Autodesk Inventor part; units mm, degrees
ref_plane "YZ Plane" through (0, 0, 0) normal (1, 0, 0) x (0, 1, 0)
ref_plane "XZ Plane" through (0, 0, 0) normal (0, 1, 0) x (-1, 0, 0)
ref_plane "XY Plane" through (0, 0, 0) normal (0, 0, 1) x (1, 0, 0)
sketch "Sketch2" plane through (0, 0, 0) normal (0, 0, 1) x (1, 0, 0)
  circle A0 centre (0, 0) radius 2.5
  circle A1 centre (0, 0) radius 6
  dimension "d12" = 5
  dimension "d13" = 12
extrude "Extrusion1" add sketch "Sketch2" along normal blind 2.5
sketch "Sketch3" plane through (0, 0, 2.5) normal (0, 0, 1) x (1, 0, 0)
  circle A0 centre (0, 0) radius 2.5
  circle A1 centre (0, 0) radius 6
  line L0 (0, 0) -> (0, -18.3723) construction
  circle A2 centre (0, -17) radius 1.5
  circle A3 centre (0, -9) radius 1.25
  line L1 (3, -5.1962) -> (3, -17)
  line L2 (-3, -17) -> (-3, -5.1962)
  line L3 (5.4814, -17) -> (-5.6867, -17) construction
  arc A4 (-3, -17) -> (3, -17) centre (0, -17) ccw
  dimension "d16" = 3
  dimension "d17" = 2.5
  dimension "d18" = 9
  dimension "d19" = 17
  dimension "d20" = 3
  dimension "d21" = 3
extrude "Extrusion2" add sketch "Sketch3" against normal blind 2.5 contours A1 L1 A4 L2
pattern_circular "Circular Pattern1" count 4 over 360 about axis through (0, 0, 0) along (0, 0, 1) of "Extrusion2"
chamfer "Chamfer1" distance 0.6 angle 45 4 edges at (-1.5, -17, 2.5) (17, -1.5, 2.5) (-17, 1.5, 2.5) (1.5, 17, 2.5)
equation "\"d21\" = d20"
properties part number "HK 2830 mounting plate"
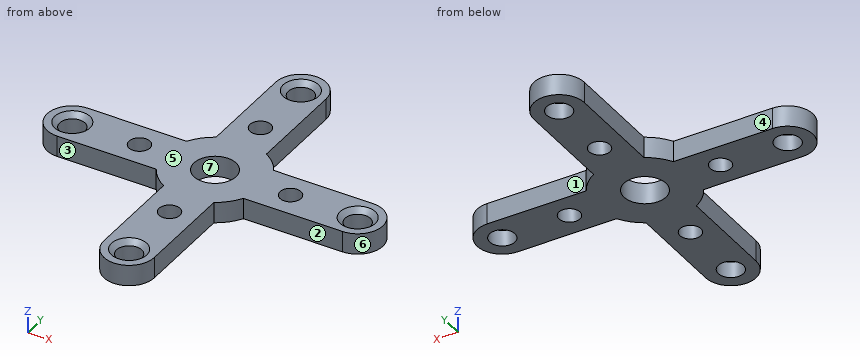
For this review, take the finished solid that the model builds, in its own axes (mm). Face numbers are marked on the shaded views. A direction names the side the tool comes from. Round coordinates to 2 decimals unless told otherwise and drop trailing zeros. Loops run counter-clockwise (first coordinate to the right, second up) from the corner with the lowest first, then second, coordinate; pieces in that order, holes last. Notation, with made-up numbers: (30.5, 20) - (78.5, 20) arc R20 ccw to (78.5, 28) - close; hole circle Ø5 at (25.5, -22). An arc over 180 degrees is marked (long way). Put each result on its own line as item: value. Start each with the question number.
1. For probe 1 along Y at (x, z) = (0, 0.65); probe 2 along Y at (x, z) = (17, 1.5), list the stretches that pass through material, from the lowest coordinate up. Write a range as [from, to].
2. Insertion check: P1, Ø1.2, axis at x = -11, z = 1.5, coming from the -Y side; P2, Ø1.2, axis at y = -11.5, z = 1.5, coming from the +X side. Each pin has a flat end and moves straight along its axis. Give the tip position at first contact, or say it passes through.
3. Mouldability with a two-part tool opening along Y and no side actions: class the marked faces 5, 6 and 7 as +Y half, -Y half, draft (parallel to the pull), parting line (faces both ways), or undercut.
4. Consider section C-C on y = -9. State the section outline as (x, z) points.
5. Consider section A-A on y = 0. State the section outline as (x, z) points.
6. For the marked faces 1, 2, 3 and 4, list the 3-axis set-ups (+Z, -Z, +X, -X, +Y, -Y) from which the entire face can be reached by the end or side of a thin tool; tool diameter is ignored.
Result sheet:
1. probe 1: [-20, -18.5], [-15.5, -10.25], [-7.75, -2.5], [2.5, 7.75], [10.25, 15.5], [18.5, 20]
1. probe 2: [-3, -1.5], [1.5, 3]
2. P1: y = -3
2. P2: x = 3
3. face 5: draft
3. face 6: parting line
3. face 7: undercut
4. outline: (-3, 0) - (-1.25, 0) - (-1.25, 2.5) - (-3, 2.5) - close; (1.25, 0) - (3, 0) - (3, 2.5) - (1.25, 2.5) - close
5. outline: (-20, 0) - (-18.5, 0) - (-18.5, 1.9) - (-19.1, 2.5) - (-20, 2.5) - close; (-15.5, 0) - (-10.25, 0) - (-10.25, 2.5) - (-14.9, 2.5) - (-15.5, 1.9) - close; (-7.75, 0) - (-2.5, 0) - (-2.5, 2.5) - (-7.75, 2.5) - close; (2.5, 0) - (7.75, 0) - (7.75, 2.5) - (2.5, 2.5) - close; (10.25, 0) - (15.5, 0) - (15.5, 1.9) - (14.9, 2.5) - (10.25, 2.5) - close; (18.5, 0) - (20, 0) - (20, 2.5) - (19.1, 2.5) - (18.5, 1.9) - close
6. face 1: +Z, -Z, +X, +Y
6. face 2: +Z, -Z, +X, -Y
6. face 3: +Z, -Z, -X, -Y
6. face 4: +Z, -Z, -X, +Y
